```python
from build123d import *

# Parameters (mm, degrees)
CROQUIS1_R              = 4.5
CROQUIS1_R_2            = 1.55
SALIENTE_EXTRUIR1_DEPTH = 1.5
CROQUIS6_R              = 1.55
CORTAR_EXTRUIR1_DEPTH   = 1.5
REDONDEO1_R             = 2


with BuildPart() as part:
    # Croquis1 → Saliente-Extruir1 (new body)
    # profile 1 of 2: a face of its own
    with BuildSketch(Plane(origin=(0, 0, 0), x_dir=(1, 0, 0), z_dir=(0, 1, 0))):
        with BuildLine():
            Line((-4.5, 13.5), (-4.5, 0))
            ThreePointArc((-4.5, 0), (0, 4.5), (4.5, 0))
            Line((4.5, 0), (4.5, 13.5))
            Line((4.5, 13.5), (-4.5, 13.5))
        make_face()
    # profile 2 of 2: a face of its own
    with BuildSketch(Plane(origin=(0, 0, 0), x_dir=(1, 0, 0), z_dir=(0, 1, 0))):
        Circle(CROQUIS1_R)
        with Locations(Location((0, 0, 0), (0, 0, 270))):
            Circle(CROQUIS1_R_2, mode=Mode.SUBTRACT)
    saliente_extruir1 = extrude(amount=SALIENTE_EXTRUIR1_DEPTH)

    # Croquis6 → Cortar-Extruir1 (cut)
    with BuildSketch(Plane(origin=(0, 1.5, 0), x_dir=(1, 0, 0), z_dir=(0, 1, 0))):
        with Locations(Location((0, 9, 0), (0, 0, 270))):
            Circle(CROQUIS6_R)
    cortar_extruir1 = extrude(amount=-CORTAR_EXTRUIR1_DEPTH, mode=Mode.SUBTRACT)

    # Simetría1: Saliente-Extruir1, Cortar-Extruir1 across plane
    add(saliente_extruir1.mirror(Plane(origin=(0, 6.75, -6.75), x_dir=(0, 0.7071067811865479, 0.7071067811865472), z_dir=(0, 0.7071067811865474, -0.7071067811865478))))
    add(cortar_extruir1.mirror(Plane(origin=(0, 6.75, -6.75), x_dir=(0, 0.7071067811865479, 0.7071067811865472), z_dir=(0, 0.7071067811865474, -0.7071067811865478))), mode=Mode.SUBTRACT)

    # Redondeo1
    redondeo1_edges = [part.edges().sort_by_distance(p)[0] for p in [
        (0, 0, -13.5),
    ]]
    fillet(redondeo1_edges, radius=REDONDEO1_R)


solid = part.part
```
Geometry: final body of the model. Coordinates: model frame, mm. Round coordinates to 2 decimals unless told otherwise and drop trailing zeros. Write each loop counter-clockwise with the first axis right and the second up, starting at its lowest first coordinate (ties: lowest second). Pieces come first, ordered by that corner, then holes.
Item 1: Section query C-C (y = 4.5). Return loops of the section in (x, z).
Item 2: Pin query (flat end, axial travel): P1, Ø2.5, axis at x = -1, y = 12.5, coming from the +Z side; P2, Ø3, axis at x = 0, y = 13.5, coming from the -Z side; P3, Ø4.5, axis at x = -2, z = -1.5, coming from the +Y side. Return the tip coordinate at first contact, or that it passes through.
Item 3: Section query D-D (x = 2.75). Return loops of the section in (y, z).
Item 4: Material intervals for L1, parallel to X at y = 0.6, z = -9; L2, parallel to Z at x = 3, y = 14.25; L3, parallel to Y at x = 3.75, z = -9.5, sorted ascending.
Item 5: Section query B-B (x = 0). Return loops of the section in (y, z), plus the area to 3 significant figures.
Item 6: Mould query, pull axis Y, two halves, no side actions, for faces 1 (the face through (0.07, 11.95, -12.76)), 2 (the face through (0.07, 2.95, -12.74)), 3 (the face through (0, 10, -12)), 4 (the face through (0, 1.5, -4)). Classes: +Y half, -Y half, draft (parallel to the pull), parting line (faces both ways), or undercut.
Item 7: Section query A-A (z = -9). Return loops of the section in (x, y), plus the area to 3 significant figures.
Completed:
1. outline: (-4.5, -13.5) - (-1.55, -13.5) - (-1.55, -12) - (-4.5, -12) - close; (1.55, -13.5) - (4.5, -13.5) - (4.5, -12) - (1.55, -12) - close
2. P1: stops at z = -12
2. P2: passes through
2. P3: stops at y = 1.5
3. outline: (0, -11.5) arc R2 ccw to (2, -13.5) - (17.06, -13.5) - (17.06, -12) - (1.5, -12) - (1.5, 3.56) - (0, 3.56) - close
4. L1: x = -4.5 to -1.55, 1.55 to 4.5
4. L2: z = -13.5 to -12
4. L3: y = 0 to 1.5
5. outline: (0, -11.5) arc R2 ccw to (2, -13.5) - (2.95, -13.5) - (2.95, -12) - (1.5, -12) - (1.5, -10.55) - (0, -10.55) - close; (0, -7.45) - (1.5, -7.45) - (1.5, -1.55) - (0, -1.55) - close; (0, 1.55) - (1.5, 1.55) - (1.5, 4.5) - (0, 4.5) - close; (6.05, -13.5) - (11.95, -13.5) - (11.95, -12) - (6.05, -12) - close; (15.05, -13.5) - (18, -13.5) - (18, -12) - (15.05, -12) - close
5. area: 32.3 mm2
6. face 1: undercut
6. face 2: undercut
6. face 3: draft
6. face 4: +Y half
7. outline: (-4.5, 0) - (-1.55, 0) - (-1.55, 1.5) - (-4.5, 1.5) - close; (1.55, 0) - (4.5, 0) - (4.5, 1.5) - (1.55, 1.5) - close
7. area: 8.85 mm2
